Autodesk Inventor part; units mm, degrees
ref_plane "C1_XY" through (0, 0, 0) normal (0, 0, 1) x (1, 0, 0)
ref_plane "C1_YZ" through (0, 0, 0) normal (1, 0, 0) x (0, 1, 0)
ref_plane "C1_ZX" through (0, 0, 0) normal (0, 1, 0) x (0, 0, 1)
sketch "Sketch_122" plane through (0, 0, 0) normal (0, 0, 1) x (1, 0, 0)
  arc A0 (-15, -13) -> (-13, -15) centre (-13, -13) ccw
  line L0 (-13, -15) -> (13, -15)
  arc A1 (13, -15) -> (15, -13) centre (13, -13) ccw
  line L1 (15, -13) -> (15, 13)
  arc A2 (15, 13) -> (13, 15) centre (13, 13) ccw
  line L2 (13, 15) -> (-13, 15)
  arc A3 (-13, 15) -> (-15, 13) centre (-13, 13) ccw
  line L3 (-15, 13) -> (-15, 4)
  line L4 (-15, 4) -> (-13, 4)
  line L5 (-13, 4) -> (-13, 8.25)
  line L6 (-13, 8.25) -> (-9.6642, 8.25)
  line L7 (-9.6642, 8.25) -> (-6, 4.5858)
  line L8 (-6, 4.5858) -> (-6, 0.5196)
  line L9 (-6, 0.5196) -> (-5.7, 0)
  line L10 (-5.7, 0) -> (-6, -0.5196)
  line L11 (-6, -0.5196) -> (-6, -4.5858)
  line L12 (-6, -4.5858) -> (-9.6642, -8.25)
  line L13 (-9.6642, -8.25) -> (-13, -8.25)
  line L14 (-13, -8.25) -> (-13, -4)
  line L15 (-13, -4) -> (-15, -4)
  line L16 (-15, -4) -> (-15, -13)
  line L17 (6, -4.5858) -> (9.6642, -8.25)
  line L18 (9.6642, -8.25) -> (13, -8.25)
  line L19 (13, -8.25) -> (13, 8.25)
  line L20 (13, 8.25) -> (9.6642, 8.25)
  line L21 (9.6642, 8.25) -> (6, 4.5858)
  line L22 (6, 4.5858) -> (6, -4.5858)
extrude "Extrusion1" add sketch "Sketch_122" against normal blind 600
sketch "Sketch2" plane through (0, 0, -600) normal (0, 0, -1) x (-1, 0, 0)
  point P0 (0, 0)
hole "Hole1" at (0, 0, -600) direction (0, 0, 1) diameter 6.8 depth 600
sketch "Sketch_173" plane through (0, 0, 0) normal (0, 0, 1) x (1, 0, 0)
  arc A0 (-9.8177, 12.6944) -> (-11.625, 9.525) centre (-11.625, 11.625) ccw
  line L0 (-11.625, 9.525) -> (-8.1108, 9.525)
  line L1 (-8.1108, 9.525) -> (-4.5858, 6)
  line L2 (-4.5858, 6) -> (4.5858, 6)
  line L3 (4.5858, 6) -> (8.1108, 9.525)
  line L4 (8.1108, 9.525) -> (11.625, 9.525)
  arc A1 (11.625, 9.525) -> (9.8177, 12.6944) centre (11.625, 11.625) ccw
  arc A2 (8.7013, 13) -> (9.8177, 12.6944) centre (9.3013, 13) ccw
  line L5 (8.7013, 13) -> (-8.7013, 13)
  arc A3 (-9.8177, 12.6944) -> (-8.7013, 13) centre (-9.3013, 13) ccw
extrude "Extrusion2" cut sketch "Sketch_173" against normal blind 600
sketch "Sketch_174" plane through (0, 0, 0) normal (0, 0, 1) x (1, 0, 0)
  arc A0 (-11.625, -9.525) -> (-9.8177, -12.6944) centre (-11.625, -11.625) ccw
  arc A1 (-8.7013, -13) -> (-9.8177, -12.6944) centre (-9.3013, -13) ccw
  line L0 (-8.7013, -13) -> (8.7013, -13)
  arc A2 (9.8177, -12.6944) -> (8.7013, -13) centre (9.3013, -13) ccw
  arc A3 (9.8177, -12.6944) -> (11.625, -9.525) centre (11.625, -11.625) ccw
  line L1 (11.625, -9.525) -> (8.1108, -9.525)
  line L2 (8.1108, -9.525) -> (4.5858, -6)
  line L3 (4.5858, -6) -> (-4.5858, -6)
  line L4 (-4.5858, -6) -> (-8.1108, -9.525)
  line L5 (-8.1108, -9.525) -> (-11.625, -9.525)
extrude "Extrusion3" cut sketch "Sketch_174" against normal blind 600
ref_plane "C1_XY" through (0, 0, 0) normal (0, 0, 1) x (1, 0, 0)
ref_plane "C1_YZ" through (0, 0, 0) normal (1, 0, 0) x (0, 1, 0)
ref_plane "C1_ZX" through (0, 0, 0) normal (0, 1, 0) x (0, 0, 1)
ref_plane "to_frame_cap1_XY" through (0, 0, 0) normal (0, 0, 1) x (1, 0, 0)
ref_plane "to_frame_cap1_YZ" through (0, 0, 0) normal (1, 0, 0) x (0, 1, 0)
ref_plane "to_frame_cap1_ZX" through (0, 0, 0) normal (0, 1, 0) x (0, 0, 1)
ref_plane "to_frame_cap2_XY" through (0, 0, -600) normal (0, 0, -1) x (1, 0, 0)
ref_plane "to_frame_cap2_YZ" through (0, 0, -600) normal (1, 0, 0) x (0, -1, 0)
ref_plane "to_frame_cap2_ZX" through (0, 0, -600) normal (0, -1, 0) x (0, 0, -1)
thread "Thread1"
thread "Thread2"
properties part number "HFSC6-3030-600" material "Aluminum 6061"
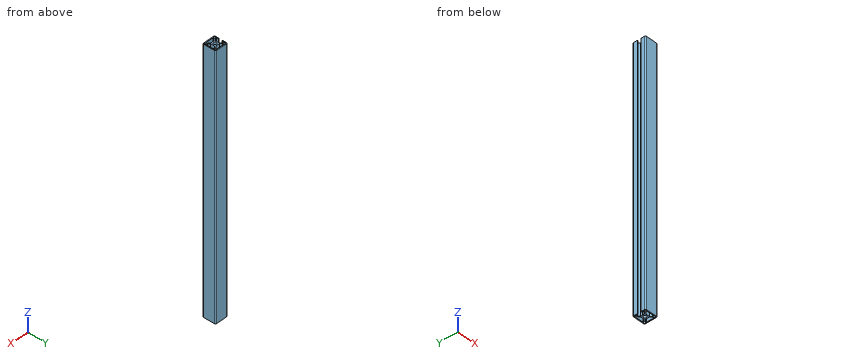
Model file for the job. Use its own axes, mm. Give positions to 0.01 mm unless a question says otherwise; leave off trailing zeros.
1) Pin check, flat tips, straight feed: pin 1 (3.5 mm diameter, centred on x = 11.63, y = 11.62, fed in from +Z); pin 2 (2 mm diameter, centred on x = -14.5, z = -290.5, fed in from +Y). Stop position of each tip, or through.
2) Wall check: probe 1 along Y at (x, z) = (0, -470); probe 2 along Y at (x, z) = (-11.75, -239); probe 3 along X at (y, z) = (-0.5, -142.5). Give the ranges that are in metal, low to high.
3) Saw through at A-A, the plane z = -353.5. Count the separate pieces of the cut face and the enclosed holes in it, then the cut area to 3 significant figures.
Computed:
1. pin 1: passes through
1. pin 2: stops at y = 14.94
2. probe 1: y = -15 to -13, -6 to -3.4, 3.4 to 6, 13 to 15
2. probe 2: y = -15 to -13.72, -9.53 to -8.25, 8.25 to 9.53, 13.72 to 15
2. probe 3: x = -5.99 to -3.36, 3.36 to 6, 13 to 15
3. separate pieces: 1
3. enclosed holes: 4
3. area: 360 mm2
